Geometry check sheet. Reference: the model listing, model coordinates, mm. A direction names the side the tool comes from. Round coordinates to 2 decimals unless told otherwise and drop trailing zeros. Write each loop counter-clockwise with the first axis right and the second up, starting at its lowest first coordinate (ties: lowest second). Pieces come first, ordered by that corner, then holes. Notation, with made-up numbers: M 33,56.5 L 85,56.5 A22 ccw 85,92.5 Z; hole C -9,-31.5 d8. An arc over 180 degrees is marked long. Answer as CSV lines item,"result". Start each with the question number.
```python
from build123d import *

# Parameters (mm, degrees)
F0_R      = 19.654875
F1_DEPTH  = 25.4
F1_FACE_R = 19.654875
F2_DEPTH  = 25.4
F3_R      = 2.265589
F4_DEPTH  = 50.8
F5_R      = 2.250211
F6_DEPTH  = 38.1


with BuildPart() as f1:
    # F0 (on Right) → F1 (new body)
    with BuildSketch(Plane.YZ):
        with Locations((0, 56.388002)):
            Circle(F0_R)
    extrude(amount=F1_DEPTH)

    # F1_face (on face) → F2 (join)
    with BuildSketch(Plane(origin=(0, 0, 56.388002), x_dir=(0, 1, 0), z_dir=(-1, 0, 0))):
        Circle(F1_FACE_R)
    extrude(amount=F2_DEPTH)

    # F3 (on Top) → F4 (join)
    with BuildSketch(Plane.XY):
        Circle(F3_R)
    extrude(amount=F4_DEPTH)

    # F5 (on Top) → F6 (join)
    with BuildSketch(Plane.XY):
        Circle(F5_R)
    extrude(amount=-F6_DEPTH)


solid = f1.part
```
1) Section check D-D, the plane z = 19. Record the cut outline in (x, y), plus the area to 3 significant figures.
2) Section check C-C, the plane z = 49. Record the cut outline in (x, y).
3) Access from +Z, -Z, +X, -X, +Y, -Y to the whole of each face (thin tool, end or side, straight path). Record for faces 1 (the flat face through (-25.4, 0, 56)), 2 (the cylindrical face through (-0.29, 2.23, -18.78)).
4) Scan lines: line 1 (Z direction, x = 11, y = -1); line 2 (Y direction, x = 2, z = -17.5); line 3 (Z direction, x = 2, y = 4.5). Record each from-to range of solid material in increasing order. Write a range as from..to.
5) Go/stop test with flat-tipped pins: pin 1 (8 mm diameter, centred on x = 1.5, y = 6, fed in from +Z); pin 2 (3 mm diameter, centred on x = -18, y = -14, fed in from -Z); pin 3 (8 mm diameter, centred on x = -16, z = 32.5, fed in from +Y). Record where each tip stops, or that it passes through.
Results:
1,outline,"C 0,0 d4.53"
1,area,"16.1 mm^2"
2,outline,"M -25.4,-18.21 L 25.4,-18.21 L 25.4,18.21 L -25.4,18.21 Z"
3,face 1,"+Z, -Z, -X, +Y, -Y"
3,face 2,"-Z"
4,line 1,"z = 36.76..76.02"
4,line 2,"y = -1.03..1.03"
4,line 3,"z = 37.26..75.52"
5,pin 1,"stops at z = 75.94"
5,pin 2,"stops at z = 41.22"
5,pin 3,"passes through"
